Geometry check sheet. Reference: the model listing, model coordinates, mm. Face numbers are marked on the shaded views. A direction names the side the tool comes from. Round coordinates to 2 decimals unless told otherwise and drop trailing zeros. Order: outer loops, then holes, each group sorted by start corner. A loop starts at its lowest first (then second) coordinate and runs counter-clockwise, first axis right, second up.
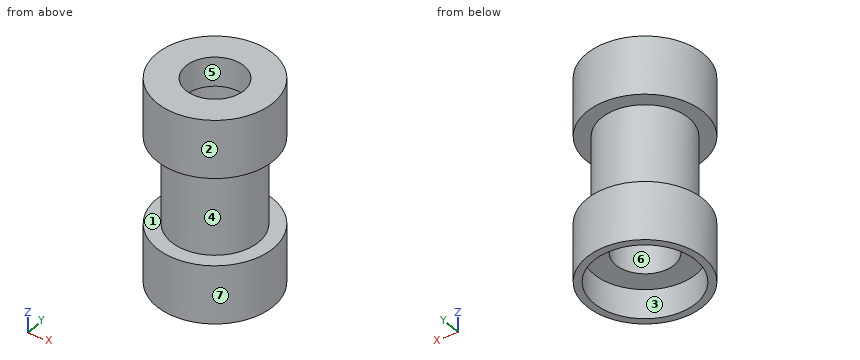
Autodesk Inventor part; units mm, degrees
ref_plane "YZ Plane" through (0, 0, 0) normal (1, 0, 0) x (0, 1, 0)
ref_plane "XZ Plane" through (0, 0, 0) normal (0, 1, 0) x (-1, 0, 0)
ref_plane "XY Plane" through (0, 0, 0) normal (0, 0, 1) x (1, 0, 0)
sketch "스케치1" plane through (0, 0, 0) normal (0, 0, 1) x (1, 0, 0)
  circle A0 centre (0, 0) radius 20
  dimension "d0" = 40
extrude "돌출1" add sketch "스케치1" along normal blind 20
sketch "스케치2" plane through (0, 0, 20) normal (0, 0, 1) x (1, 0, 0)
  circle A0 centre (0, 0) radius 15
  dimension "d3" = 30
extrude "돌출2" add sketch "스케치2" along normal blind 30
sketch "스케치3" plane through (0, 0, 50) normal (0, 0, 1) x (1, 0, 0)
  circle A0 centre (0, 0) radius 20
  dimension "d6" = 40
extrude "돌출3" add sketch "스케치3" along normal blind 20
sketch "스케치4" plane through (0, 0, 0) normal (0, 0, -1) x (-1, 0, 0)
  circle A0 centre (0, 0) radius 17.5
  dimension "d9" = 35
extrude "돌출4" cut sketch "스케치4" against normal blind 10
sketch "스케치5" plane through (0, 0, 10) normal (0, 0, -1) x (-1, 0, 0)
  circle A0 centre (0, 0) radius 10
  dimension "d12" = 20
extrude "돌출5" cut sketch "스케치5" against normal blind 15
sketch "스케치6" plane through (0, 0, 25) normal (0, 0, -1) x (-1, 0, 0)
  circle A0 centre (0, 0) radius 5
  dimension "d15" = 10
extrude "돌출6" cut sketch "스케치6" against normal blind 20
sketch "스케치9" plane through (0, 0, 45) normal (0, 0, -1) x (-1, 0, 0)
  circle A0 centre (0, 0) radius 12.5
  dimension "d22" = 25
extrude "돌출8" cut sketch "스케치9" against normal blind 15
sketch "스케치10" plane through (0, 0, 60) normal (0, 0, -1) x (-1, 0, 0)
  circle A0 centre (0, 0) radius 10
  dimension "d25" = 20
extrude "돌출9" cut sketch "스케치10" against normal up to next
properties part number "기본 투상 연습1"
(1) Depth check by flat-ended pin: P1, Ø8, axis at x = 12.5, z = 40, coming from the -Y side; P2, Ø23, axis at x = 0, y = 0, coming from the +Z side; P3, Ø9, axis at x = 0, y = 0, coming from the +Z side; P4, Ø6, axis at x = -0.5, y = -2.5, coming from the +Z side. Enter the tip coordinate at first touch or a pass-through.
Returned:
P1: stops at y = -12.36
P2: stops at z = 70
P3: passes through
P4: stops at z = 45
(2) Sectioned sample at D-D, the plane x = 13.5. Record the cut outline in (y, z).
Returned:
outline: (-14.76, 0) - (-11.14, 0) - (-11.14, 10) - (11.14, 10) - (11.14, 0) - (14.76, 0) - (14.76, 20) - (6.54, 20) - (6.54, 50) - (14.76, 50) - (14.76, 70) - (-14.76, 70) - (-14.76, 50) - (-6.54, 50) - (-6.54, 20) - (-14.76, 20) - close
(3) Draft check along X on the marked faces 1, 2 and 3. Enter one of: released by +X, released by -X, zero draft, split by the parting line, or undercut.
Returned:
face 1: zero draft
face 2: split by the parting line
face 3: undercut
(4) Material ranges on line 1 (X direction, y = -0.5, z = 46); line 2 (Y direction, x = 0, z = 13.5); line 3 (Y direction, x = 0, z = 51), recorded low to high.
Returned:
line 1: x = -14.99 to -12.49, 12.49 to 14.99
line 2: y = -20 to -10, 10 to 20
line 3: y = -20 to -12.5, 12.5 to 20
(5) Set-up check for the marked faces 4, 5, 6 and 7: record each of +Z, -Z, +X, -X, +Y, -Y from which the full face is reachable in a straight line by a thin tool's end or side.
Returned:
face 4: none
face 5: +Z
face 6: -Z
face 7: +Z, -Z
(6) Sectioned sample at C-C, the plane z = 65. Record the cut outline in (x, y), and give its area (3 significant figures).
Returned:
outline: circle Ø40 at (0, 0); hole circle Ø20 at (0, 0)
area: 942 mm2
